from build123d import *

# Parameters (mm, degrees)
SKETCH1_R           = 12.7
SKETCH1_R_2         = 5.3975
BOSS_EXTRUDE1_DEPTH = 7.62
SKETCH2_R           = 14.224
SKETCH2_R_2         = 5.3975
BOSS_EXTRUDE2_DEPTH = 1.27
CUT_EXTRUDE1_DEPTH  = 9.89
CUT_EXTRUDE2_DEPTH  = 2.27
FILLET1_R           = 0.762


with BuildPart() as part:
    # Sketch1 → Boss-Extrude1 (new body)
    with BuildSketch(Plane.XY):
        Circle(SKETCH1_R)
        Circle(SKETCH1_R_2, mode=Mode.SUBTRACT)
    extrude(amount=BOSS_EXTRUDE1_DEPTH)

    # Sketch2 → Boss-Extrude2 (add)
    with BuildSketch(Plane.XY.offset(7.62)):
        Circle(SKETCH2_R)
        Circle(SKETCH2_R_2, mode=Mode.SUBTRACT)
    extrude(amount=BOSS_EXTRUDE2_DEPTH)

    # Sketch3 → Cut-Extrude1 (cut, through all)
    with BuildSketch(Plane(origin=(0, 0, 0), x_dir=(-1, 0, 0), z_dir=(0, 0, -1))):
        with BuildLine():
            Line((-1.905, 14.224), (1.905, 14.224))
            Line((1.905, 14.224), (1.905, -11.141309797))
            ThreePointArc((1.905, -11.141309797), (0, -11.303), (-1.905, -11.141309797))
            Line((-1.905, -11.141309797), (-1.905, 14.224))
        make_face()
    extrude(amount=-CUT_EXTRUDE1_DEPTH, mode=Mode.SUBTRACT)

    # Sketch4 → Cut-Extrude2 (cut, through all)
    with BuildSketch(Plane(origin=(0, 0, 7.62), x_dir=(-1, 0, 0), z_dir=(0, 0, -1))):
        with BuildLine():
            Line((-1.905, -14.224), (-1.905, -12.556312158))
            ThreePointArc((-1.905, -12.556312158), (0, -12.7), (1.905, -12.556312158))
            Line((1.905, -12.556312158), (1.905, -14.224))
            Line((1.905, -14.224), (-1.905, -14.224))
        make_face()
    extrude(amount=-CUT_EXTRUDE2_DEPTH, mode=Mode.SUBTRACT)

    # Fillet1
    fillet1_edges = [part.edges().sort_by_distance(p)[0] for p in [
        (1.905, -11.141309797, 4.445),
        (-1.905, -11.141309797, 4.445),
    ]]
    fillet(fillet1_edges, radius=FILLET1_R)


solid = part.part
Design review of the part built by this model. Coordinates are the model's own, in mm. A direction names the side the tool comes from. Round coordinates to 2 decimals unless told otherwise and drop trailing zeros. Loops run counter-clockwise (first coordinate to the right, second up) from the corner with the lowest first, then second, coordinate; pieces in that order, holes last. Notation, with made-up numbers: (-32.75, -29.75) -> (-14.75, -29.75) arc R17 cw to (-14.75, 0.25) -> close; hole circle Ø3 at (17, -21). An arc over 180 degrees is marked (long way). Use one line per item in the form item = value. Start each with the question number.
Q1. We need section A-A on y = 0. Give the boundary of the cut face in (x, z).
Q2. Draft analysis for pull direction X (two halves, no side actions). For faces 5 (the face through (14.22, -0.29, 8.25)), 6 (the face through (13, 2, 7.62)), 7 (the face through (-1.905, -13, 8)), 8 (the face through (-5.397, 0.091, 4.383)), state which applies: +X half, -X half, draft (parallel to the pull), parting line (faces both ways), or undercut.
Q3. We need section B-B on z = 4.5. Give the boundary of the cut face in (x, y) (1 decimal).
Q4. For pin 1 Ø5 at (y, z) = (-11, 5.5) entering from -X; pin 2 Ø4.5 at (y, z) = (8.5, 4.5) entering from +X; pin 3 Ø1.5 at (x, z) = (2.5, 6.5) entering from +Y, all flat-tipped, find the tip position at first contact; note any pin that passes through.
Q5. We need section D-D on x = 0. Give the boundary of the cut face in (y, z).
Q6. We need section C-C on y = -9.75. Give the boundary of the cut face in (x, z) (3 decimals), then the cut area to 3 significant figures.
Q7. Machinability: for faces 1 (the face through (-13, 0, 7.62)), 2 (the face through (5.397, -0.091, 4.383)), 3 (the face through (-1.905, -8, 4)), 4 (the face through (1.905, -13, 8)), which of the approach directions +Z, -Z, +X, -X, +Y, -Y give a long, thin tool a straight path to every point of the face, cutting with its end or side? Answer none if there is none.
Q8. Wall thickness on line 1 along X through (y, z) = (-0.5, 1.5); line 2 along Y through (x, z) = (-2.25, 8.5); line 3 along X through (y, z) = (1.25, 1.5): over which ranges is each line inside the solid? List them lowest first. Write a range as [from, to].
Calculated:
q1.outline = (-14.22, 7.62) -> (-12.7, 7.62) -> (-12.7, 0) -> (-5.4, 0) -> (-5.4, 8.89) -> (-14.22, 8.89) -> close; (5.4, 0) -> (12.7, 0) -> (12.7, 7.62) -> (14.22, 7.62) -> (14.22, 8.89) -> (5.4, 8.89) -> close
q2.face_5 = +X half
q2.face_6 = draft
q2.face_7 = undercut
q2.face_8 = undercut
q3.outline = (-1.9, -10.5) -> (-1.9, -5.1) arc R5.4 cw to (-1.9, 5.1) -> (-1.9, 12.6) arc R12.7 ccw (long way) to (1.9, 12.6) -> (1.9, 5.1) arc R5.4 cw to (1.9, -5.1) -> (1.9, -10.5) arc R0.8 cw to (1.2, -11.2) arc R11.3 cw to (-1.2, -11.2) arc R0.8 cw to start
q4.pin_1 = -10.43
q4.pin_2 = 11.06
q4.pin_3 = 12.56
q5.outline = (-12.7, 0) -> (-11.3, 0) -> (-11.3, 8.89) -> (-12.7, 8.89) -> close
q6.outline = (-10.357, 7.62) -> (-8.138, 7.62) -> (-8.138, 0) -> (-1.905, 0) -> (-1.905, 8.89) -> (-10.357, 8.89) -> close; (1.905, 0) -> (8.138, 0) -> (8.138, 7.62) -> (10.357, 7.62) -> (10.357, 8.89) -> (1.905, 8.89) -> close
q6.area = 116 mm²
q7.face_1 = -Z, -X
q7.face_2 = +Z, -Z
q7.face_3 = +Z, -Z, +Y
q7.face_4 = +Z, -Z, -Y
q8.line_1 = [-12.69, -5.37], [5.37, 12.69]
q8.line_2 = [-14.04, -4.91], [4.91, 14.04]
q8.line_3 = [-12.64, -5.25], [5.25, 12.64]
